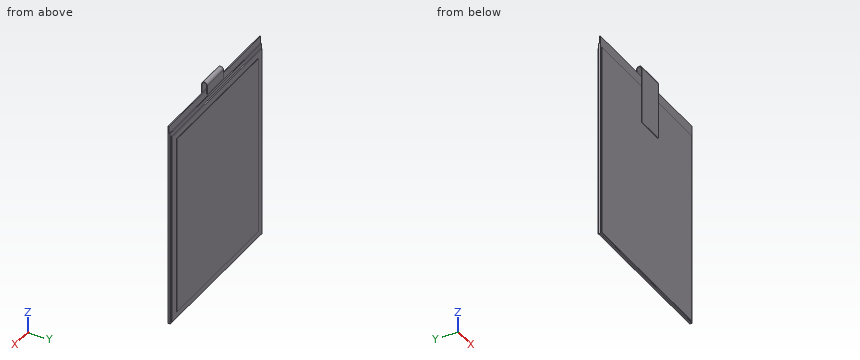
```python
from build123d import *

# Parameters (mm, degrees)
SKETCH1_W           = 31
SKETCH1_H           = 41.46
BOSS_EXTRUDE1_DEPTH = 0.2
SKETCH2_W           = 31
SKETCH2_H           = 40
BOSS_EXTRUDE2_DEPTH = 0.2
SKETCH3_W           = 30.4
SKETCH3_H           = 38.96
BOSS_EXTRUDE3_DEPTH = 0.23
SKETCH4_W           = 30.4
SKETCH4_H           = 38.96
BOSS_EXTRUDE4_DEPTH = 0.115
BOSS_EXTRUDE5_DEPTH = 2.75
SKETCH7_W           = 27.6
SKETCH7_H           = 36.36
BOSS_EXTRUDE6_DEPTH = 0.1


with BuildPart() as part:
    # Sketch1 → Boss-Extrude1 (new body)
    with BuildSketch(Plane(origin=(0, 0, 0), x_dir=(1, 0, 0), z_dir=(0, 1, 0))):
        Rectangle(SKETCH1_W, SKETCH1_H)
    extrude(amount=BOSS_EXTRUDE1_DEPTH)

    # Sketch2 → Boss-Extrude2 (add)
    with BuildSketch(Plane(origin=(0, 0.2, 0), x_dir=(1, 0, 0), z_dir=(0, 1, 0))):
        with Locations((0, 0.73)):
            Rectangle(SKETCH2_W, SKETCH2_H)
    extrude(amount=BOSS_EXTRUDE2_DEPTH)

    # Sketch3 → Boss-Extrude3 (add)
    with BuildSketch(Plane(origin=(0, 0.4, 0), x_dir=(1, 0, 0), z_dir=(0, 1, 0))):
        with Locations((0, 0.95)):
            Rectangle(SKETCH3_W, SKETCH3_H)
    extrude(amount=BOSS_EXTRUDE3_DEPTH)

    # Sketch4 → Boss-Extrude4 (add)
    with BuildSketch(Plane.XZ):
        with Locations((0, -0.95)):
            Rectangle(SKETCH4_W, SKETCH4_H)
    extrude(amount=BOSS_EXTRUDE4_DEPTH)

    # Sketch5 → Boss-Extrude5 (add, symmetric)
    with BuildSketch(Plane(origin=(0, 0, 0), x_dir=(0, 0, -1), z_dir=(1, 0, 0))):
        with BuildLine():
            Line((-20.73, 0.2), (-21.53, 0.2))
            ThreePointArc((-21.53, 0.2), (-21.98, -0.25), (-21.53, -0.7))
            Line((-21.53, -0.7), (-10.13, -0.7))
            Line((-10.13, -0.7), (-10.13, -0.8))
            Line((-10.13, -0.8), (-21.53, -0.8))
            ThreePointArc((-21.53, -0.8), (-22.08, -0.25), (-21.53, 0.3))
            Line((-21.53, 0.3), (-19.73, 0.3))
            Line((-19.73, 0.3), (-19.73, 0.2))
            Line((-19.73, 0.2), (-20.73, 0.2))
        make_face()
    extrude(amount=BOSS_EXTRUDE5_DEPTH, both=True)

    # Sketch7 → Boss-Extrude6 (add)
    with BuildSketch(Plane(origin=(0, 0.63, 0), x_dir=(1, 0, 0), z_dir=(0, 1, 0))):
        with Locations((0, 0.95)):
            Rectangle(SKETCH7_W, SKETCH7_H)
    extrude(amount=BOSS_EXTRUDE6_DEPTH)


solid = part.part
```
The model under review builds one solid part; all positions refer to its coordinate system, in mm. Coordinates: 2 decimals unless noted, no trailing zeros. Write each loop counter-clockwise with the first axis right and the second up, starting at its lowest first coordinate (ties: lowest second). Pieces come first, ordered by that corner, then holes. Notation, with made-up numbers: (60, -2.75) -> (92, -2.75) arc R29 ccw to (92, 22.25) -> close; hole circle Ø11 at (46.5, -6.5). An arc over 180 degrees is marked (long way). One line per item, written item: value. Start each with the question number.
Q1. Add section B-B, the plane x = -7. Give the boundary of the cut face in (y, z) (3 decimals).
Q2. Add section A-A, the plane z = 18. Give the boundary of the cut face in (x, y) (3 decimals).
Q3. To check wall thickness, follow probe 1 along Y at (x, z) = (-1.5, -4.5) (3 decimals); probe 2 along Z at (x, y) = (-7.5, 0.35); probe 3 along Y at (x, z) = (14.5, -13) (3 decimals). State the ranges of each line that lie inside material, in increasing order.
Q4. Add section C-C, the plane z = 11.5. Give the boundary of the cut face in (x, y) (3 decimals), then the cut area to 3 significant figures.
Q5. Add section D-D, the plane z = 0. Give the boundary of the cut face in (x, y) (3 decimals).
Q6. Clearance check with flat-ended pins moving along their axes: P1, Ø0.9, axis at x = 0.5, z = 21, coming from the +Y side; P2, Ø4, axis at x = -7, z = -2.5, coming from the -Y side (3 decimals); P3, Ø15.5, axis at x = 5, z = 4, coming from the -Y side; P4, Ø0.9, axis at y = -0.5, z = 19, coming from the -X side. State where each tip first meets the part, or that it passes through.
Response:
1. outline: (-0.115, -20.43) -> (0, -20.43) -> (0, -20.73) -> (0.4, -20.73) -> (0.4, -20.43) -> (0.63, -20.43) -> (0.63, -19.13) -> (0.73, -19.13) -> (0.73, 17.23) -> (0.63, 17.23) -> (0.63, 18.53) -> (0.4, 18.53) -> (0.4, 19.27) -> (0.2, 19.27) -> (0.2, 20.73) -> (0, 20.73) -> (0, 18.53) -> (-0.115, 18.53) -> close
2. outline: (-15.5, 0) -> (-15.2, 0) -> (-15.2, -0.115) -> (15.2, -0.115) -> (15.2, 0) -> (15.5, 0) -> (15.5, 0.4) -> (15.2, 0.4) -> (15.2, 0.63) -> (-15.2, 0.63) -> (-15.2, 0.4) -> (-15.5, 0.4) -> close; (-2.75, -0.8) -> (2.75, -0.8) -> (2.75, -0.7) -> (-2.75, -0.7) -> close
3. probe 1: -0.115 to 0.73
3. probe 2: -20.73 to 19.27
3. probe 3: -0.115 to 0.63
4. outline: (-15.5, 0) -> (-15.2, 0) -> (-15.2, -0.115) -> (15.2, -0.115) -> (15.2, 0) -> (15.5, 0) -> (15.5, 0.4) -> (15.2, 0.4) -> (15.2, 0.63) -> (13.8, 0.63) -> (13.8, 0.73) -> (-13.8, 0.73) -> (-13.8, 0.63) -> (-15.2, 0.63) -> (-15.2, 0.4) -> (-15.5, 0.4) -> close; (-2.75, -0.8) -> (2.75, -0.8) -> (2.75, -0.7) -> (-2.75, -0.7) -> close
4. area: 26.2 mm²
5. outline: (-15.5, 0) -> (-15.2, 0) -> (-15.2, -0.115) -> (15.2, -0.115) -> (15.2, 0) -> (15.5, 0) -> (15.5, 0.4) -> (15.2, 0.4) -> (15.2, 0.63) -> (13.8, 0.63) -> (13.8, 0.73) -> (-13.8, 0.73) -> (-13.8, 0.63) -> (-15.2, 0.63) -> (-15.2, 0.4) -> (-15.5, 0.4) -> close
6. P1: y = 0.3
6. P2: y = -0.115
6. P3: y = -0.8
6. P4: x = -2.75
